Can you work these out from the drawing? Everything is in mm from the part's minimum corner. Round coordinates to 2 decimals unless told otherwise and drop trailing zeros. Order: outer loops, then holes, each group sorted by start corner. A loop starts at its lowest first (then second) coordinate and runs counter-clockwise, first axis right, second up. Notation, with made-up numbers: (18.25, 9) - (58.25, 9) arc R6 cw to (58.25, 16) - close; hole circle Ø7 at (46.25, 16.5). An arc over 180 degrees is marked (long way). Answer as a JSON object with one key per item and string values.
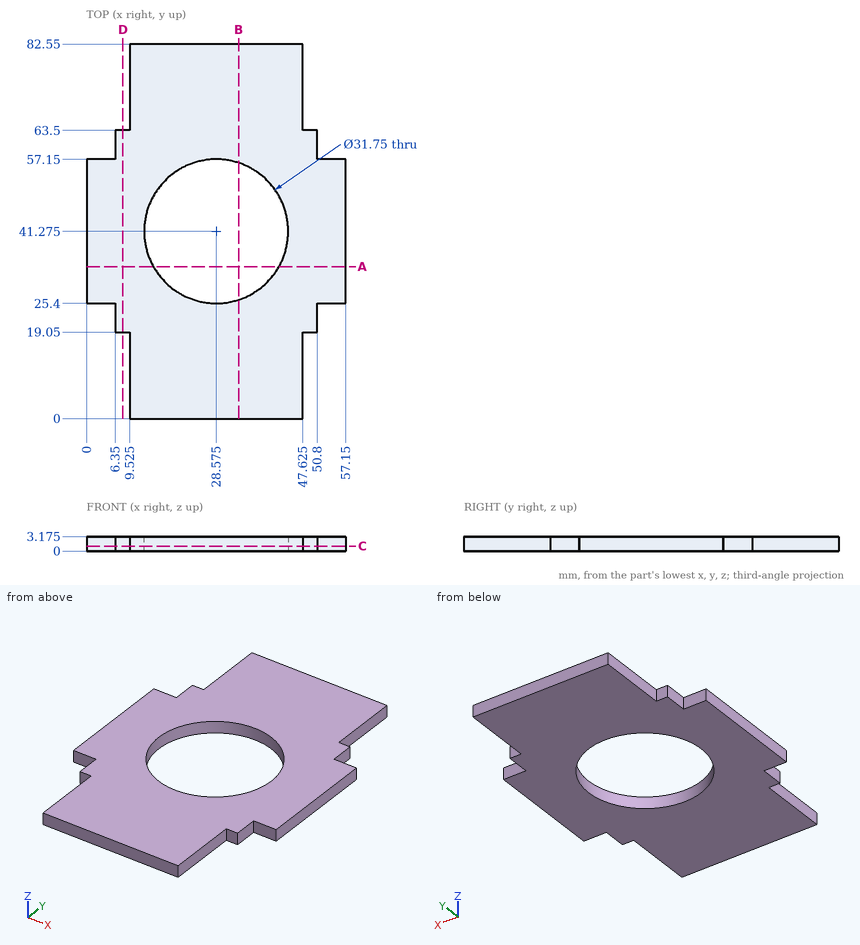
1. Imagine slicing it at C-C (z = 1.1). List the corners of the cut face in (x, y) for me (3 decimals), plus the area to 3 significant figures.
Responses:
{"outline": "(0, 25.4) - (6.35, 25.4) - (6.35, 19.05) - (9.525, 19.05) - (9.525, 0) - (47.625, 0) - (47.625, 19.05) - (50.8, 19.05) - (50.8, 25.4) - (57.15, 25.4) - (57.15, 57.15) - (50.8, 57.15) - (50.8, 63.5) - (47.625, 63.5) - (47.625, 82.55) - (9.525, 82.55) - (9.525, 63.5) - (6.35, 63.5) - (6.35, 57.15) - (0, 57.15) - close; hole circle Ø31.75 at (28.575, 41.275)", "area": "3,040 mm2"}
2. For P1, Ø1.6, axis at y = 8.5, z = 2, coming from the -X side (3 decimals); P2, Ø1, axis at x = 54.5, z = 1.5, coming from the -Y side; P3, Ø1, axis at x = 3, z = 2, coming from the +Y side, each with a flat end and sliding along its axis, tell me the tip position at first contact or that it passes through.
Responses:
{"P1": "x = 9.525", "P2": "y = 25.4", "P3": "y = 57.15"}
3. Imagine slicing it at A-A (y = 33.5). List the corners of the cut face in (x, z) for me (3 decimals), plus the area to 3 significant figures.
Responses:
{"outline": "(0, 0) - (14.734, 0) - (14.734, 3.175) - (0, 3.175) - close; (42.416, 0) - (57.15, 0) - (57.15, 3.175) - (42.416, 3.175) - close", "area": "93.6 mm2"}
4. If I drill on L1, parallel to X at y = 19, z = 0.8 (3 decimals); L2, parallel to X at y = 46.5, z = 2.65; L3, parallel to Y at x = 40, z = 2.6, over which ranges is the centre line in solid material (lowest first)? Write a range as [from, to].
Responses:
{"L1": "[9.525, 47.625]", "L2": "[0, 13.58], [43.57, 57.15]", "L3": "[0, 30.25], [52.3, 82.55]"}
5. Imagine slicing it at B-B (x = 33.5). List the corners of the cut face in (y, z) for me (3 decimals), plus the area to 3 significant figures.
Responses:
{"outline": "(0, 0) - (26.183, 0) - (26.183, 3.175) - (0, 3.175) - close; (56.367, 0) - (82.55, 0) - (82.55, 3.175) - (56.367, 3.175) - close", "area": "166 mm2"}
6. Imagine slicing it at D-D (x = 8). List the corners of the cut face in (y, z) for me (3 decimals), plus the area to 3 significant figures.
Responses:
{"outline": "(19.05, 0) - (63.5, 0) - (63.5, 3.175) - (19.05, 3.175) - close", "area": "141 mm2"}
